Design review of the part built by this model. Coordinates are the model's own, in mm. Face numbers are marked on the shaded views. A direction names the side the tool comes from. Round coordinates to 2 decimals unless told otherwise and drop trailing zeros. Write each loop counter-clockwise with the first axis right and the second up, starting at its lowest first coordinate (ties: lowest second). Pieces come first, ordered by that corner, then holes. Notation, with made-up numbers: (15.5, 79) -> (72.5, 79) arc R5 ccw to (72.5, 88) -> close; hole circle Ø7 at (-22, -14). An arc over 180 degrees is marked (long way). One line per question, with ' | ' between items. Start each with the question number.
1) Insertion check: pin 1 Ø3 at (x, y) = (7, -11) entering from -Z; pin 2 Ø7 at (y, z) = (16.5, 13.5) entering from +X; pin 3 Ø15 at (y, z) = (11, 18) entering from -X; pin 4 Ø1 at (x, y) = (11, 1.5) entering from +Z. Each pin has a flat end and moves straight along its axis. Give the tip position at first contact, or say it passes through.
2) For probe 1 along Y at (x, z) = (0, 9.25); probe 2 along Y at (x, z) = (-12, 16.5); probe 3 along Z at (x, y) = (17, -10), list the stretches that pass through material, from the lowest coordinate up.
3) For the marked faces 1, 2, 3, 4 and 5, list the 3-axis set-ups (+Z, -Z, +X, -X, +Y, -Y) from which the entire face can be reached by the end or side of a thin tool; tool diameter is ignored.
4) Mouldability with a two-part tool opening along X and no side actions: class the marked faces 6, 7, 8 and 9 as +X half, -X half, draft (parallel to the pull), parting line (faces both ways), or undercut.
5) Consider section B-B (x = 0). Give the boundary of the cut face in (y, z).
6) Consider section A-A (y = -13.75). Give the boundary of the cut face in (x, z).
7) Consider section D-D (x = 6). Give the boundary of the cut face in (y, z).
8) Consider section C-C (z = 20.75). Give the boundary of the cut face in (x, y), then the cut area to 3 significant figures.
```python
from build123d import *

# Parameters (mm, degrees)
SKETCH_W        = 40
SKETCH_H        = 40
SKETCH_R        = 2.25
PAD_DEPTH       = 25
SKETCH001_W     = 40
SKETCH001_H     = 13
POCKET_DEPTH    = 20
SKETCH002_W     = 6
SKETCH002_H     = 42
POCKET001_DEPTH = 20


with BuildPart() as part:
    # Sketch → Pad (new body)
    with BuildSketch(Plane.XY):
        Rectangle(SKETCH_W, SKETCH_H)
        with Locations((0, 13.75)):
            Circle(SKETCH_R, mode=Mode.SUBTRACT)
        with Locations((0, -13.75)):
            Circle(SKETCH_R, mode=Mode.SUBTRACT)
        with BuildLine():
            ThreePointArc((-4.999983, 4.5), (-9.499983, 9e-06), (-5, -4.5))
            Line((-5, -4.5), (5, -4.5))
            ThreePointArc((5, -4.5), (9.499983, 9e-06), (4.999983, 4.5))
            Line((-4.999983, 4.5), (4.999983, 4.5))
        make_face(mode=Mode.SUBTRACT)
    extrude(amount=PAD_DEPTH)

    # Sketch001 → Pocket (cut)
    with BuildSketch(Plane.XY.offset(25)):
        Rectangle(SKETCH001_W, SKETCH001_H)
    extrude(amount=-POCKET_DEPTH, mode=Mode.SUBTRACT)

    # Sketch002 → Pocket001 (cut)
    with BuildSketch(Plane.XY.offset(25)):
        with Locations((-18, 0)):
            Rectangle(SKETCH002_W, SKETCH002_H)
        with Locations((18, 0)):
            Rectangle(SKETCH002_W, SKETCH002_H)
    extrude(amount=-POCKET001_DEPTH, mode=Mode.SUBTRACT)


solid = part.part
```
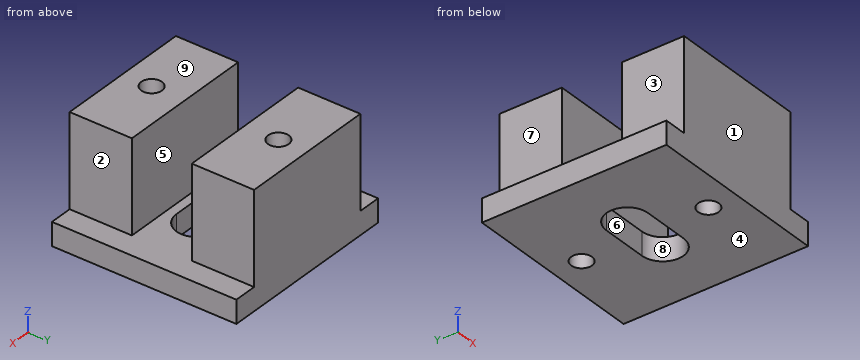
From the geometry:
1) pin 1: stops at z = 0 | pin 2: stops at x = 15 | pin 3: stops at x = -15 | pin 4: stops at z = 5
2) probe 1: y = -20 to -16, -11.5 to -6.5, 6.5 to 11.5, 16 to 20 | probe 2: y = -20 to -6.5, 6.5 to 20 | probe 3: z = 0 to 5
3) face 1: +Z, -Z, +X, -X, -Y | face 2: +Z, +X, +Y, -Y | face 3: +Z, -X, +Y, -Y | face 4: -Z, +X, -X, +Y, -Y | face 5: +Z, +X, -X
4) face 6: undercut | face 7: -X half | face 8: undercut | face 9: draft
5) outline: (-20, 0) -> (-16, 0) -> (-16, 25) -> (-20, 25) -> close; (-11.5, 0) -> (-4.5, 0) -> (-4.5, 5) -> (-6.5, 5) -> (-6.5, 25) -> (-11.5, 25) -> close; (4.5, 0) -> (11.5, 0) -> (11.5, 25) -> (6.5, 25) -> (6.5, 5) -> (4.5, 5) -> close; (16, 0) -> (20, 0) -> (20, 25) -> (16, 25) -> close
6) outline: (-20, 0) -> (-2.25, 0) -> (-2.25, 25) -> (-15, 25) -> (-15, 5) -> (-20, 5) -> close; (2.25, 0) -> (20, 0) -> (20, 5) -> (15, 5) -> (15, 25) -> (2.25, 25) -> close
7) outline: (-20, 0) -> (-4.39, 0) -> (-4.39, 5) -> (-6.5, 5) -> (-6.5, 25) -> (-20, 25) -> close; (4.39, 0) -> (20, 0) -> (20, 25) -> (6.5, 25) -> (6.5, 5) -> (4.39, 5) -> close
8) outline: (-15, -20) -> (15, -20) -> (15, -6.5) -> (-15, -6.5) -> close; (-15, 6.5) -> (15, 6.5) -> (15, 20) -> (-15, 20) -> close; hole circle Ø4.5 at (0, -13.75); hole circle Ø4.5 at (0, 13.75) | area: 778 mm2
